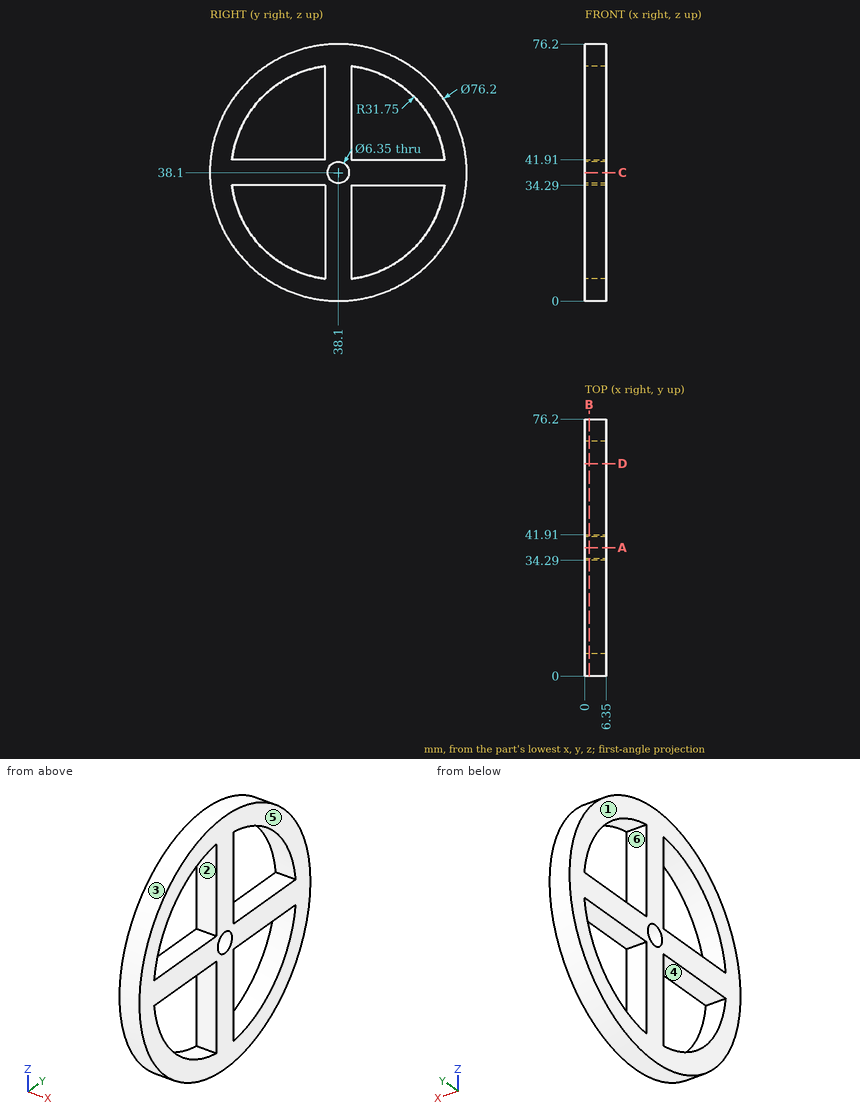
Geometry check sheet. Reference: drawing and pictorial views, mm from the part's lowest x, y, z. A direction names the side the tool comes from. Give positions to 0.01 mm unless a question says otherwise; leave off trailing zeros. Order: outer loops, then holes, each group sorted by start corner. A loop starts at its lowest first (then second) coordinate and runs counter-clockwise, first axis right, second up. Notation, with made-up numbers: M 68,54 L 90,54 A16 ccw 90,81 Z; hole C 35.25,-15.75 d11. An arc over 180 degrees is marked long. Answer as a JSON object with one key per item and string values. Group by question number.
1) Scan lines: line 1 along Z through (x, y) = (2.5, 38.1) (3 decimals); line 2 along Z through (x, y) = (1.5, 66.5); line 3 along Y through (x, z) = (5, 9.5). Record each from-to range of solid material in increasing order. Write a range as [from, to].
2) Cross-section at D-D (y = 63). Enter the section's corners in (x, z), then the cut area to 3 significant figures.
3) Access from +Z, -Z, +X, -X, +Y, -Y to the whole of each face (thin tool, end or side, straight path). Record for the marked faces 5 and 6.
4) Depth check by flat-ended pin: pin 1 Ø3 at (x, y) = (3.5, 56) entering from -Z; pin 2 Ø1.9 at (x, y) = (4.5, 19.5) entering from -Z; pin 3 Ø1 at (x, z) = (2.5, 11) entering from -Y. Enter the tip coordinate at first touch or a pass-through.
5) Mould release check, pull along Z, two halves, no side actions. Record for the marked faces 1, 2, 3 and 4: released by +Z, released by -Z, zero draft, split by the parting line, or undercut.
6) Cross-section at A-A (y = 38.1). Enter the section's corners in (x, z) (3 decimals).
7) Cross-section at B-B (x = 1.25). Enter the section's corners in (y, z) (3 decimals).
Result sheet:
{
 "1": {"line 1": "z = [0, 34.925], [41.275, 76.2]", "line 2": "z = [12.7, 23.9], [34.29, 41.91], [52.3, 63.5]", "line 3": "y = [12.93, 24.31], [34.29, 41.91], [51.89, 63.27]"},
 "2": {"outline": "M 0,9.26 L 6.35,9.26 L 6.35,18.4 L 0,18.4 Z; M 0,34.29 L 6.35,34.29 L 6.35,41.91 L 0,41.91 Z; M 0,57.8 L 6.35,57.8 L 6.35,66.94 L 0,66.94 Z", "area": "164 mm2"},
 "3": {"face 5": "+Z, -Z, +X, +Y, -Y", "face 6": "+X, -X"},
 "4": {"pin 1": "stops at z = 3.71", "pin 2": "stops at z = 4.33", "pin 3": "stops at y = 10.82"},
 "5": {"face 1": "zero draft", "face 2": "undercut", "face 3": "split by the parting line", "face 4": "undercut"},
 "6": {"outline": "M 0,0 L 6.35,0 L 6.35,34.925 L 0,34.925 Z; M 0,41.275 L 6.35,41.275 L 6.35,76.2 L 0,76.2 Z"},
 "7": {"outline": "C 38.1,38.1 d76.2; hole M 6.579,34.29 A31.75 ccw 34.29,6.579 L 34.29,34.29 Z; hole M 6.579,41.91 L 34.29,41.91 L 34.29,69.621 A31.75 ccw Z; hole C 38.1,38.1 d6.35; hole M 41.91,6.579 A31.75 ccw 69.621,34.29 L 41.91,34.29 Z; hole M 41.91,41.91 L 69.621,41.91 A31.75 ccw 41.91,69.621 Z"}
}
